Model file for the job. Use its own axes, mm. A direction names the side the tool comes from. Coordinates: 2 decimals unless noted, no trailing zeros. Write each loop counter-clockwise with the first axis right and the second up, starting at its lowest first coordinate (ties: lowest second). Pieces come first, ordered by that corner, then holes. Notation, with made-up numbers: (34, 4.5) - (68, 4.5) arc R21 cw to (68, 8.5) - close; hole circle Ø1 at (35, 38.5). An arc over 180 degrees is marked (long way). Put each result on its own line as item: value. Start each with the question number.
1. Saw through at B-B, the plane z = 1. Write the cut outline in (x, y).
2. Pull direction Y, two halves, no side cores. Call faces 6 (the face through (7.8, -0.6, 1.2)), 7 (the face through (-6, 0, -15.25)), 8 (the face through (-5.76, 1.28, 8.97)): released by +Y, released by -Y, zero draft, split by the parting line, or undercut.
3. Saw through at C-C, the plane y = 2. Write the cut outline in (x, z), plus the area to 3 significant figures.
4. Saw through at A-A, the plane x = -19.4. Write the cut outline in (y, z).
5. Drill centre lines: L1, parallel to Y at x = -19.4, z = 1.5; L2, parallel to Z at x = -12, y = 1.75; L3, parallel to Z at x = 8.5, y = 1.25. Where is each one in solid material? Low to high. Write a range as from..to.
6. Drop flat-ended pins along their axis: P1, Ø1.2, axis at x = -19.4, y = 0, coming from the +Z side; P2, Ø6, axis at y = 0, z = -6.5, coming from the -X side; P3, Ø4, axis at x = -18.5, y = 2, coming from the +Z side; P4, Ø1.5, axis at x = -19, y = 2, coming from the -Z side. Give the stop position or say it passes through.
7. Which spindle directions (+Z, -Z, +X, -X, +Y, -Y) get a long thin tool onto all of the face, cutting with end or side? Do faces 1 (the face through (-18, 0, 2.43)), 2 (the face through (4, 5, 7)), 3 (the face through (-16.7, 0, -8)), 4 (the face through (5.9, 0, 5)), 5 (the face through (5, -5, 7)). Say none if no direction does.
```python
from build123d import *

# Parameters (mm, degrees)
F0_W     = 5
F0_H     = 11.8
F0_R     = 1
F1_DEPTH = 2.43
F2_DEPTH = 7
F3_DEPTH = 11
F4_DEPTH = 15.25


with BuildPart() as f1:
    # F0 (on Top) → F1 (new body)
    with BuildSketch(Plane.XY):
        with Locations((-19.2, 0)):
            Rectangle(F0_W, F0_H)
        with Locations((-19.4, 0)):
            Circle(F0_R, mode=Mode.SUBTRACT)
        with BuildLine():
            Line((6e-09, 5.9), (-16.7, 5.9))
            Line((-16.7, 5.9), (-16.7, -5.9))
            Line((-16.7, -5.9), (1.1e-09, -5.9))
            ThreePointArc((1.1e-09, -5.9), (-5.9, 2.4e-09), (6e-09, 5.9))
        make_face()
        with BuildLine():
            ThreePointArc((5.9, 0), (4.1719300111, 4.1719300069), (6e-09, 5.9))
            ThreePointArc((6e-09, 5.9), (-5.9, 2.4e-09), (1.1e-09, -5.9))
            ThreePointArc((1.1e-09, -5.9), (4.1719300094, -4.1719300086), (5.9, 0))
        make_face()
        with BuildLine():
            Line((5.9, 5.9), (6e-09, 5.9))
            ThreePointArc((6e-09, 5.9), (4.1719300111, 4.1719300069), (5.9, 0))
            Line((5.9, 0), (5.9, 5.9))
        make_face()
        with BuildLine():
            Line((5.9, -5.9), (5.9, 0))
            ThreePointArc((5.9, 0), (4.1719300094, -4.1719300086), (1.1e-09, -5.9))
            Line((1.1e-09, -5.9), (5.9, -5.9))
        make_face()
        Polygon((10.9, 5.9), (5.9, 5.9), (5.9, 0), (5.9, -5.9), (10.9, -5.9), align=None)
        with Locations((8.6, 0)):
            Circle(F0_R, mode=Mode.SUBTRACT)
    extrude(amount=F1_DEPTH)

    # F0 (on Top) → F2 (join)
    with BuildSketch(Plane.XY):
        with BuildLine():
            Line((6e-09, 5.9), (-16.7, 5.9))
            Line((-16.7, 5.9), (-16.7, -5.9))
            Line((-16.7, -5.9), (1.1e-09, -5.9))
            ThreePointArc((1.1e-09, -5.9), (-5.9, 2.4e-09), (6e-09, 5.9))
        make_face()
        with BuildLine():
            ThreePointArc((5.9, 0), (4.1719300111, 4.1719300069), (6e-09, 5.9))
            ThreePointArc((6e-09, 5.9), (-5.9, 2.4e-09), (1.1e-09, -5.9))
            ThreePointArc((1.1e-09, -5.9), (4.1719300094, -4.1719300086), (5.9, 0))
        make_face()
        with BuildLine():
            Line((5.9, -5.9), (5.9, 0))
            ThreePointArc((5.9, 0), (4.1719300094, -4.1719300086), (1.1e-09, -5.9))
            Line((1.1e-09, -5.9), (5.9, -5.9))
        make_face()
        with BuildLine():
            Line((5.9, 5.9), (6e-09, 5.9))
            ThreePointArc((6e-09, 5.9), (4.1719300111, 4.1719300069), (5.9, 0))
            Line((5.9, 0), (5.9, 5.9))
        make_face()
    extrude(amount=F2_DEPTH)

    # F0 (on Top) → F3 (join)
    with BuildSketch(Plane.XY):
        with BuildLine():
            ThreePointArc((5.9, 0), (4.1719300111, 4.1719300069), (6e-09, 5.9))
            ThreePointArc((6e-09, 5.9), (-5.9, 2.4e-09), (1.1e-09, -5.9))
            ThreePointArc((1.1e-09, -5.9), (4.1719300094, -4.1719300086), (5.9, 0))
        make_face()
    extrude(amount=F3_DEPTH)

    # F0 (on Top) → F4 (join)
    with BuildSketch(Plane.XY):
        with BuildLine():
            Line((6e-09, 5.9), (-16.7, 5.9))
            Line((-16.7, 5.9), (-16.7, -5.9))
            Line((-16.7, -5.9), (1.1e-09, -5.9))
            ThreePointArc((1.1e-09, -5.9), (-5.9, 2.4e-09), (6e-09, 5.9))
        make_face()
        with BuildLine():
            ThreePointArc((5.9, 0), (4.1719300111, 4.1719300069), (6e-09, 5.9))
            ThreePointArc((6e-09, 5.9), (-5.9, 2.4e-09), (1.1e-09, -5.9))
            ThreePointArc((1.1e-09, -5.9), (4.1719300094, -4.1719300086), (5.9, 0))
        make_face()
        with BuildLine():
            Line((5.9, -5.9), (5.9, 0))
            ThreePointArc((5.9, 0), (4.1719300094, -4.1719300086), (1.1e-09, -5.9))
            Line((1.1e-09, -5.9), (5.9, -5.9))
        make_face()
        with BuildLine():
            Line((5.9, 5.9), (6e-09, 5.9))
            ThreePointArc((6e-09, 5.9), (4.1719300111, 4.1719300069), (5.9, 0))
            Line((5.9, 0), (5.9, 5.9))
        make_face()
    extrude(amount=-F4_DEPTH)


solid = f1.part
```
Final values:
1. outline: (-21.7, -5.9) - (10.9, -5.9) - (10.9, 5.9) - (-21.7, 5.9) - close; hole circle Ø2 at (-19.4, 0); hole circle Ø2 at (8.6, 0)
2. face 6: undercut
2. face 7: zero draft
2. face 8: split by the parting line
3. outline: (-21.7, 0) - (-16.7, 0) - (-16.7, -15.25) - (5.9, -15.25) - (5.9, 0) - (10.9, 0) - (10.9, 2.43) - (5.9, 2.43) - (5.9, 7) - (5.55, 7) - (5.55, 11) - (-5.55, 11) - (-5.55, 7) - (-16.7, 7) - (-16.7, 2.43) - (-21.7, 2.43) - close
3. area: 572 mm²
4. outline: (-5.9, 0) - (-1, 0) - (-1, 2.43) - (-5.9, 2.43) - close; (1, 0) - (5.9, 0) - (5.9, 2.43) - (1, 2.43) - close
5. L1: y = -5.9..-1, 1..5.9
5. L2: z = -15.25..7
5. L3: z = 0..2.43
6. P1: passes through
6. P2: stops at x = -16.7
6. P3: stops at z = 7
6. P4: stops at z = 0
7. face 1: +Z, -X, +Y, -Y
7. face 2: +Z, +X, +Y
7. face 3: -Z, -X, +Y, -Y
7. face 4: +Z, +X, +Y, -Y
7. face 5: +Z, +X, -Y
